Source: CAD feature listing. Evaluate the final solid. Frame: model axes, mm. Give positions to 0.01 mm unless a question says otherwise; leave off trailing zeros. Order: outer loops, then holes, each group sorted by start corner. A loop starts at its lowest first (then second) coordinate and runs counter-clockwise, first axis right, second up.
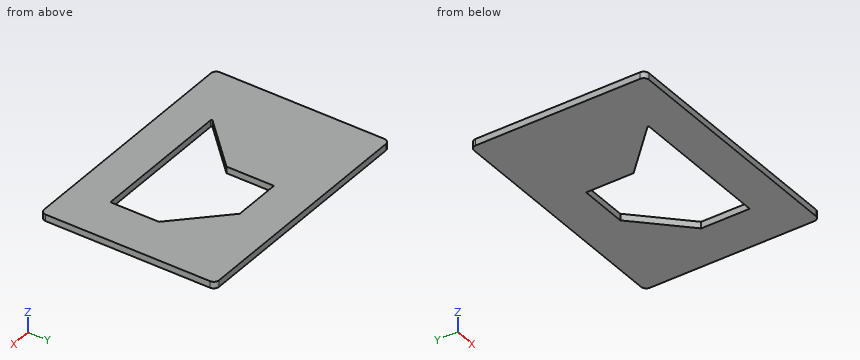
```python
from build123d import *

# Parameters (mm, degrees)
F1_DEPTH = 6.35
F3_DEPTH = 25.4
F5_DEPTH = 25.4


with BuildPart() as f1:
    # F0 (on Top) → F1 (new body)
    with BuildSketch(Plane.XY):
        with BuildLine():
            Line((113.9825, 84.1375), (-113.9825, 84.1375))
            ThreePointArc((-113.9825, 84.1375), (-117.574602, 82.649602), (-119.0625, 79.0575))
            Line((-119.0625, 79.0575), (-119.0625, -79.0575))
            ThreePointArc((-119.0625, -79.0575), (-117.574602, -82.649602), (-113.9825, -84.1375))
            Line((-113.9825, -84.1375), (113.9825, -84.1375))
            ThreePointArc((113.9825, -84.1375), (117.574602, -82.649602), (119.0625, -79.0575))
            Line((119.0625, -79.0575), (119.0625, 79.0575))
            ThreePointArc((119.0625, 79.0575), (117.574602, 82.649602), (113.9825, 84.1375))
        make_face()
    extrude(amount=F1_DEPTH)

    # F2 (on face) → F3 (cut)
    with BuildSketch(Plane.XY.offset(6.35)):
        Polygon((-15.246781, -1.136219), (-60.148061, -46.0375), (74.6125, -46.0375), (74.6125, -1.0795), (29.711219, 43.821781), (-15.246781, 43.821781), align=None)
    extrude(amount=-F3_DEPTH, mode=Mode.SUBTRACT)

    # F4 (on face) → F5 (cut)
    with BuildSketch(Plane.XY.offset(6.35)):
        with BuildLine():
            ThreePointArc((75.8825, -0.879601), (75.822563, -0.578276), (75.651876, -0.322825))
            Line((75.651876, -0.322825), (30.467895, 44.861156))
            ThreePointArc((30.467895, 44.861156), (30.212444, 45.031843), (29.911119, 45.091781))
            Line((29.911119, 45.091781), (-15.729381, 45.091781))
            ThreePointArc((-15.729381, 45.091781), (-16.286156, 44.861156), (-16.516781, 44.304381))
            Line((-16.516781, 44.304381), (-16.516781, -0.284016))
            ThreePointArc((-16.516781, -0.284016), (-16.576718, -0.585341), (-16.747405, -0.840792))
            Line((-16.747405, -0.840792), (-61.869937, -45.963324))
            ThreePointArc((-61.869937, -45.963324), (-62.040623, -46.821425), (-61.313161, -47.3075))
            Line((-61.313161, -47.3075), (75.0951, -47.3075))
            ThreePointArc((75.0951, -47.3075), (75.651876, -47.076876), (75.8825, -46.5201))
            Line((75.8825, -46.5201), (75.8825, -0.879601))
        make_face()
    extrude(amount=-F5_DEPTH, mode=Mode.SUBTRACT)


solid = f1.part
```
1) Section query A-A, the plane z = 3.75. Return the cut outline in (x, y).
Report:
outline: (-119.06, -79.06) arc R5.08 ccw to (-113.98, -84.14) - (113.98, -84.14) arc R5.08 ccw to (119.06, -79.06) - (119.06, 79.06) arc R5.08 ccw to (113.98, 84.14) - (-113.98, 84.14) arc R5.08 ccw to (-119.06, 79.06) - close; hole (-61.87, -45.96) arc R0.79 ccw to (-61.31, -47.31) - (75.1, -47.31) arc R0.79 ccw to (75.88, -46.52) - (75.88, -0.88) arc R0.79 ccw to (75.65, -0.32) - (30.47, 44.86) arc R0.79 ccw to (29.91, 45.09) - (-15.73, 45.09) arc R0.79 ccw to (-16.52, 44.3) - (-16.52, -0.28) arc R0.79 cw to (-16.75, -0.84) - close
2) Material intervals for L1, parallel to Y at x = 14, z = 5; L2, parallel to Y at x = -42, z = 3.5; L3, parallel to X at y = 19, z = 4.5, sorted ascending.
Report:
L1: y = -84.14 to -47.31, 45.09 to 84.14
L2: y = -84.14 to -47.31, -26.09 to 84.14
L3: x = -119.06 to -16.52, 56.33 to 119.06
3) Section query C-C, the plane y = -9. Return the cut outline in (x, z), and give its area (3 significant figures).
Report:
outline: (-119.06, 0) - (-24.91, 0) - (-24.91, 6.35) - (-119.06, 6.35) - close; (75.88, 0) - (119.06, 0) - (119.06, 6.35) - (75.88, 6.35) - close
area: 872 mm2
4) Section query B-B, the plane x = -1.5. Return the cut outline in (y, z).
Report:
outline: (-84.14, 0) - (-47.31, 0) - (-47.31, 6.35) - (-84.14, 6.35) - close; (45.09, 0) - (84.14, 0) - (84.14, 6.35) - (45.09, 6.35) - close
5) Pin query (flat end, axial travel): pin 1 (12 mm diameter, centred on x = -7, y = 34, fed in from -Z). Return the tip coordinate at first contact, or that it passes through.
Report:
pin 1: passes through
